Geometry check sheet. Reference: the model listing, model coordinates, mm. Give positions to 0.01 mm unless a question says otherwise; leave off trailing zeros. Write each loop counter-clockwise with the first axis right and the second up, starting at its lowest first coordinate (ties: lowest second). Pieces come first, ordered by that corner, then holes.
(1) Cross-section at D-D (x = 38.5). Record the boundary of the cut face in (y, z).
(2) Cross-section at A-A (z = 25). Record the boundary of the cut face in (x, y).
(3) Mould release check, pull along Z, two halves, no side actions. Record for faces 1 (the flat face through (23.1, -45.8, 50)), 2 (the cylindrical face through (23.175, -48.964, 44.964)), 3 (the flat face through (23.1, -45.8, 0)), 4 (the cylindrical face through (27.752, -47.465, 10.357)): +Z half, -Z half, draft (parallel to the pull), parting line (faces both ways), or undercut.
(4) Cross-section at B-B (x = 23.5). Record the boundary of the cut face in (y, z), and give its area (3 significant figures).
(5) Cross-section at C-C (z = 47). Record the boundary of the cut face in (x, y), and give its area (3 significant figures).
(6) Thickness scan on line 1 along Y through (x, z) = (23.5, 5.5); line 2 along X through (y, z) = (-47.5, 5.5); line 3 along X through (y, z) = (-48.7, 26). Record the ranges inside material, lowest first.
```python
from build123d import *

# Parameters (mm, degrees)
ESQUISSE1_W             = 58
ESQUISSE1_H             = 5
BOSS_EXTRU_1_DEPTH      = 50
ESQUISSE2_R             = 15
ENL_V_MAT_EXTRU_1_DEPTH = 6
ESQUISSE5_R             = 1.5
ENL_V_MAT_EXTRU_4_DEPTH = 51


with BuildPart() as part:
    # Esquisse1 → Boss.-Extru.1 (new body)
    with BuildSketch(Plane.XY):
        with Locations((23.5, -47.5)):
            Rectangle(ESQUISSE1_W, ESQUISSE1_H)
    extrude(amount=BOSS_EXTRU_1_DEPTH)

    # Esquisse2 → Enlèv. mat.-Extru.1 (cut, through all)
    with BuildSketch(Plane(origin=(0, -45, 0), x_dir=(-1, 0, 0), z_dir=(0, 1, 0))):
        with Locations((-24.5, 25)):
            Circle(ESQUISSE2_R)
    extrude(amount=-ENL_V_MAT_EXTRU_1_DEPTH, mode=Mode.SUBTRACT)

    # Esquisse5 → Enlèv. mat.-Extru.4 (cut, through all)
    with BuildSketch(Plane.XY.offset(50)):
        with Locations((23.5, -47.5)):
            Circle(ESQUISSE5_R)
    extrude(amount=-ENL_V_MAT_EXTRU_4_DEPTH, mode=Mode.SUBTRACT)


solid = part.part
```
Reply:
1. outline: (-50, 0) - (-45, 0) - (-45, 19.61) - (-50, 19.61) - close; (-50, 30.39) - (-45, 30.39) - (-45, 50) - (-50, 50) - close
2. outline: (-5.5, -50) - (9.5, -50) - (9.5, -45) - (-5.5, -45) - close; (39.5, -50) - (52.5, -50) - (52.5, -45) - (39.5, -45) - close
3. face 1: +Z half
3. face 2: draft
3. face 3: -Z half
3. face 4: undercut
4. outline: (-50, 0) - (-49, 0) - (-49, 10.03) - (-50, 10.03) - close; (-50, 39.97) - (-49, 39.97) - (-49, 50) - (-50, 50) - close; (-46, 0) - (-45, 0) - (-45, 10.03) - (-46, 10.03) - close; (-46, 39.97) - (-45, 39.97) - (-45, 50) - (-46, 50) - close
4. area: 40.1 mm2
5. outline: (-5.5, -50) - (52.5, -50) - (52.5, -45) - (-5.5, -45) - close; hole circle Ø3 at (23.5, -47.5)
5. area: 283 mm2
6. line 1: y = -50 to -49, -46 to -45
6. line 2: x = -5.5 to 22, 25 to 52.5
6. line 3: x = -5.5 to 9.53, 39.47 to 52.5
